Verification items for the finished model (mm, model axes). A direction names the side the tool comes from. Coordinates: 2 decimals unless noted, no trailing zeros. Order: outer loops, then holes, each group sorted by start corner. A loop starts at its lowest first (then second) coordinate and runs counter-clockwise, first axis right, second up. Notation, with made-up numbers: M -26.75,-19 L 14.25,-19 A29 ccw 14.25,9 Z; hole C -9,0.5 d8. An arc over 180 degrees is marked long. Write item = value, one per line.
```python
from build123d import *

# Parameters (mm, degrees)
F0_R     = 40
F0_R_2   = 9
F1_DEPTH = 3
F2_DEPTH = 18
F3_DEPTH = 25
F4_R     = 3
F5_R     = 1.614
F6_DEPTH = 40
F7_DEPTH = 5


with BuildPart() as f1:
    # F0 (on Top) → F1 (new body)
    with BuildSketch(Plane.XY):
        Circle(F0_R)
        with Locations((-21.6333586723, -12.0185324922)):
            Circle(F0_R_2, mode=Mode.SUBTRACT)
        with Locations((0.1144621056, -25.0672250986)):
            Circle(F0_R_2, mode=Mode.SUBTRACT)
        with Locations((21.6333605349, -12.247457169)):
            Circle(F0_R_2, mode=Mode.SUBTRACT)
        with Locations((-21.6506350946, 12.5)):
            Circle(F0_R_2, mode=Mode.SUBTRACT)
        with BuildLine():
            ThreePointArc((-12.5, 0), (0, 12.5), (12.5, 0))
            Line((12.5, 0), (5, 0))
            ThreePointArc((5, 0), (0, -5), (-5, 0))
            Line((-5, 0), (-12.5, 0))
        make_face(mode=Mode.SUBTRACT)
        with Locations((21.6333605349, 12.934230268)):
            Circle(F0_R_2, mode=Mode.SUBTRACT)
        with Locations((0.1144621056, 25.0672250986)):
            Circle(F0_R_2, mode=Mode.SUBTRACT)
        with BuildLine():
            Line((5, 0), (12.5, 0))
            ThreePointArc((12.5, 0), (0, 12.5), (-12.5, 0))
            Line((-12.5, 0), (-5, 0))
            ThreePointArc((-5, 0), (0, 5), (5, 0))
        make_face()
    extrude(amount=F1_DEPTH)

    # F0 (on Top) → F2 (join)
    with BuildSketch(Plane.XY):
        with BuildLine():
            Line((5, 0), (12.5, 0))
            ThreePointArc((12.5, 0), (0, 12.5), (-12.5, 0))
            Line((-12.5, 0), (-5, 0))
            ThreePointArc((-5, 0), (0, 5), (5, 0))
        make_face()
    extrude(amount=F2_DEPTH)

    # F0 (on Top) → F3 (cut)
    with BuildSketch(Plane.XY):
        Circle(F0_R)
        with Locations((-21.6333586723, -12.0185324922)):
            Circle(F0_R_2, mode=Mode.SUBTRACT)
        with Locations((0.1144621056, -25.0672250986)):
            Circle(F0_R_2, mode=Mode.SUBTRACT)
        with Locations((21.6333605349, -12.247457169)):
            Circle(F0_R_2, mode=Mode.SUBTRACT)
        with Locations((-21.6506350946, 12.5)):
            Circle(F0_R_2, mode=Mode.SUBTRACT)
        with BuildLine():
            ThreePointArc((-12.5, 0), (0, 12.5), (12.5, 0))
            Line((12.5, 0), (5, 0))
            ThreePointArc((5, 0), (0, -5), (-5, 0))
            Line((-5, 0), (-12.5, 0))
        make_face(mode=Mode.SUBTRACT)
        with Locations((21.6333605349, 12.934230268)):
            Circle(F0_R_2, mode=Mode.SUBTRACT)
        with Locations((0.1144621056, 25.0672250986)):
            Circle(F0_R_2, mode=Mode.SUBTRACT)
    extrude(amount=-F3_DEPTH, mode=Mode.SUBTRACT)

    # F4
    f4_edges = [f1.edges().sort_by_distance(p)[0] for p in [
        (0, 12.5, 3),
    ]]
    fillet(f4_edges, radius=F4_R)

    # F5 (on Right) → F6 (cut)
    with BuildSketch(Plane.YZ):
        with Locations((0, 13.645786792)):
            Circle(F5_R)
    extrude(amount=-F6_DEPTH, mode=Mode.SUBTRACT)

    # F7 (add): a face of the model
    f7_faces = [f1.faces().sort_by_distance(p)[0] for p in [
        (0, 5.9114693148, 18),
    ]]
    extrude(f7_faces, amount=F7_DEPTH)


solid = f1.part
```
Item 1: Scan lines: L1, parallel to Y at x = 27.5, z = 2; L2, parallel to Y at x = -22, z = 1; L3, parallel to Z at x = 10.5, y = -24.5. Record each from-to range of solid material in increasing order. Write a range as from..to.
Report:
L1 = -29.05..-19.07, -5.42..6.11, 19.76..29.05
L2 = -33.41..-21.01, -3.03..3.51, 21.49..33.41
L3 = 0..3
Item 2: Tool access check on faces 1 (the cylindrical face through (-8.562, 1.614, 13.61)), 2 (the flat face through (-1, -8, 0)), 3 (the cylindrical face through (0.275, 12.497, 14.381)), 4 (the cylindrical face through (0.651, 4.957, 11.339)), 5 (the flat face through (9, 0, 13)). Record the directions out of +Z, -Z, +X, -X, +Y, -Y that give a thin tool (end or side, any length) a straight path to the whole face; none if there is none.
Report:
face_1 = -X, -Y
face_2 = -Z, +X, -X, +Y, -Y
face_3 = +Z, +Y
face_4 = +Z, -Z
face_5 = +Z, +X, -X, -Y
Item 3: Release check for a two-part mould opening along X. For faces 6 (the flat face through (-9, 0, 7)), 7 (the cylindrical face through (-8.67, -39.05, 1.48)), 8 (the cylindrical face through (15, 19.017, 1.479)) record: pulls with the +X half, pulls with the -X half, needs draft (parallel to the pull), parting line crosses it, or undercut.
Report:
face_6 = needs draft
face_7 = parting line crosses it
face_8 = undercut
Item 4: Sectioned sample at A-A, the plane x = 0. Enter the section's corners in (y, z), then the cut area to 3 significant figures.
Report:
outline = M -40,0 L -34.07,0 L -34.07,3 L -40,3 Z; M -16.07,0 L -5,0 L -5,3 L -16.07,3 Z; M 5,0 L 16.07,0 L 16.07,3 L 15.5,3 A3 cw 12.5,6 L 12.5,23 L 5,23 Z; M 34.07,0 L 40,0 L 40,3 L 34.07,3 Z
area = 254 mm^2
Item 5: Sectioned sample at D-D, the plane y = -7. Enter the section's corners in (x, z).
Report:
outline = M -39.38,0 L -29.1,0 L -29.1,3 L -39.38,3 Z; M -14.16,0 L 14.32,0 L 14.32,3 L -14.16,3 Z; M 28.95,0 L 39.38,0 L 39.38,3 L 28.95,3 Z
Item 6: Sectioned sample at B-B, the plane y = -29.5. Enter the section's corners in (x, z), then the cut area to 3 significant figures.
Report:
outline = M -27.01,0 L -7.72,0 L -7.72,3 L -27.01,3 Z; M 7.95,0 L 27.01,0 L 27.01,3 L 7.95,3 Z
area = 115 mm^2
Item 7: Sectioned sample at C-C, the plane x = 16.5. Enter the section's corners in (y, z), then the cut area to 3 significant figures.
Report:
outline = M -36.44,0 L -19.64,0 L -19.64,3 L -36.44,3 Z; M -4.85,0 L 5.54,0 L 5.54,3 L -4.85,3 Z; M 20.33,0 L 36.44,0 L 36.44,3 L 20.33,3 Z
area = 130 mm^2
Item 8: Gauge pin test, flat ends, axial feed: pin 1 (14.5 mm diameter, centred on x = 21.63, y = -12.25, fed in from -Z); pin 2 (8 mm diameter, centred on x = -5, z = 13.5, fed in from +Y); pin 3 (7 mm diameter, centred on x = -10, z = 6, fed in from -Y); pin 4 (8.5 mm diameter, centred on x = 10, z = 9, fed in from -Y). Record the tip position at first contact, or that the pin passes through.
Report:
pin_1 = through
pin_2 = 12.46
pin_3 = -39.15
pin_4 = 0
